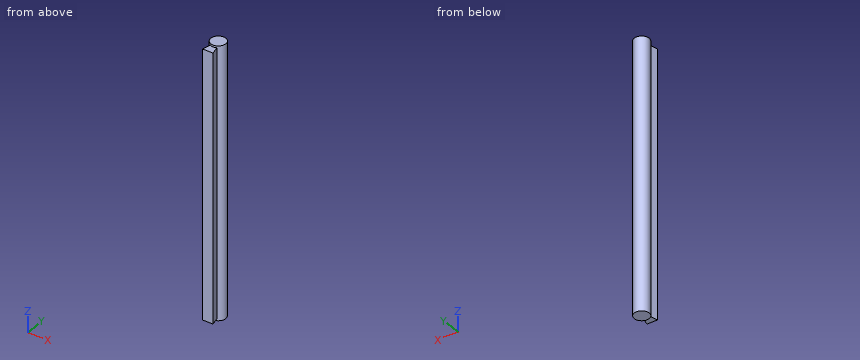
```python
from build123d import *

# Parameters (mm, degrees)
SKETCH1_R           = 12.7
BASE_EXTRUDE_DEPTH  = 457.2
BOSS_EXTRUDE1_DEPTH = 450.85


with BuildPart() as part:
    # Sketch1 → Base-Extrude (new body)
    with BuildSketch(Plane.XY):
        Circle(SKETCH1_R)
    extrude(amount=BASE_EXTRUDE_DEPTH)

    # Sketch2 → Boss-Extrude1 (add)
    with BuildSketch(Plane.XY.offset(3.175)):
        with BuildLine():
            Line((-8.763, -25.4), (8.763, -25.4))
            Line((8.763, -25.4), (5.7689526, -11.314114455))
            ThreePointArc((5.7689526, -11.314114455), (0, -12.7), (-5.7689526, -11.314114455))
            Line((-5.7689526, -11.314114455), (-8.763, -25.4))
        make_face()
    extrude(amount=BOSS_EXTRUDE1_DEPTH)


solid = part.part
```
The listing builds one solid part. Answer for the finished solid, in the listing's coordinates (mm). Give positions to 0.01 mm unless a question says otherwise; leave off trailing zeros. Write each loop counter-clockwise with the first axis right and the second up, starting at its lowest first coordinate (ties: lowest second). Pieces come first, ordered by that corner, then holes. Notation, with made-up numbers: (-8, 13) - (-2, 13) arc R26 cw to (-2, 42) - close; hole circle Ø6 at (81, -0.5). An arc over 180 degrees is marked (long way). Use one line per item in the form item = value. Start each with the question number.
1) Consider line 1 along Z through (x, y) = (3.75, -21) (3 decimals); line 2 along X through (y, z) = (-0.5, 240); line 3 along Y through (x, z) = (1.25, 36). Determine where each line is inside the solid, lowest interval first. Write a range as from..to.
2) Find section A-A on z = 344. Determine the outline of the cut face in (x, y), plus the area to 3 significant figures.
3) Flat-ended cylindrical pins translate along their axes: pin 1 Ø7 at (x, y) = (-3, -19) entering from +Z (3 decimals); pin 2 Ø8 at (y, z) = (7.5, 339.5) entering from -X; pin 3 Ø6 at (y, z) = (-14, 144.5) entering from +X. Find the tip coordinate at first contact, or state that the pin passes through.
Geometry results:
q1.line_1 = 3.175..454.025
q1.line_2 = -12.69..12.69
q1.line_3 = -25.4..12.64
q2.outline = (-8.76, -25.4) - (8.76, -25.4) - (5.77, -11.31) arc R12.7 ccw (long way) to (-5.77, -11.31) - close
q2.area = 701 mm2
q3.pin_1 = 454.025
q3.pin_2 = -12.21
q3.pin_3 = 6.98
